Geometry: final body of the model. Coordinates: model frame, mm. A direction names the side the tool comes from. Coordinates: 2 decimals unless noted, no trailing zeros. Order: outer loops, then holes, each group sorted by start corner. A loop starts at its lowest first (then second) coordinate and runs counter-clockwise, first axis right, second up. Notation, with made-up numbers: M 1,51.5 L 19,51.5 A29 ccw 19,81.5 Z; hole C 0,-9 d11. An arc over 180 degrees is marked long. Use CSV: the item, a comma, the result in double quotes. Start each with the question number.
Q1. Access query for faces 1 (the face through (36.1, 4, -8)), 2 (the face through (40, 4, -3.1)), 3 (the face through (41, 3.3, -8)). Directions: +Z, -Z, +X, -X, +Y, -Y. A direction counts if a zero-diameter tool reaches every point of the face in a straight line with its end or side. Return the directions, or none.
Q2. First-contact query: P1, Ø0.5, axis at x = 41, y = 4, coming from the -Z side; P2, Ø6, axis at x = 14, z = -13.5, coming from the +Y side; P3, Ø1.1, axis at x = 40, y = 3.5, coming from the +Z side. Flat tips, straight axial feed; report the tip coordinate or a pass-through.
Q3. Section query C-C, the plane y = 3.85. Output: boundary loops of the cut face in (x, z), and give its area (3 significant figures).
Q4. Section query B-B, the plane x = 29. Output: boundary loops of the cut face in (y, z), and give its area (3 significant figures).
Q5. Section query A-A, the plane z = -8.5. Output: boundary loops of the cut face in (x, y).
Q6. Ray query, probe 1 along X at (y, z) = (0.2, -3.5); probe 2 along Y at (x, z) = (3, -5); probe 3 along Y at (x, z) = (39.5, -12.5). Return the intervals inside material, ascending.
from build123d import *

# Parameters (mm, degrees)
SKETCH_1_W      = 38.6
SKETCH_1_H      = 16.2
EXTRUDE_1_DEPTH = 3.3
SKETCH_2_W      = 2.5
SKETCH_2_H      = 10
EXTRUDE_2_DEPTH = 1
SKETCH_3_W      = 10
SKETCH_3_H      = 1
EXTRUDE_3_DEPTH = 5.5


with BuildPart() as part:
    # 草图1 → 凸台-拉伸1 (new body)
    with BuildSketch(Plane(origin=(0, 0, 0), x_dir=(1, 0, 0), z_dir=(0, 1, 0))):
        with Locations((19.3, 8.1)):
            Rectangle(SKETCH_1_W, SKETCH_1_H)
    extrude(amount=EXTRUDE_1_DEPTH)

    # 草图2 → 凸台-拉伸2 (add)
    with BuildSketch(Plane(origin=(0, 3.3, 0), x_dir=(1, 0, 0), z_dir=(0, 1, 0))):
        with Locations((37.35, 8.1)):
            Rectangle(SKETCH_2_W, SKETCH_2_H)
    extrude(amount=EXTRUDE_2_DEPTH)

    # 草图3 → 凸台-拉伸3 (add)
    with BuildSketch(Plane(origin=(38.6, 0, 0), x_dir=(0, 0, -1), z_dir=(1, 0, 0))):
        with Locations((8.1, 3.8)):
            Rectangle(SKETCH_3_W, SKETCH_3_H)
    extrude(amount=EXTRUDE_3_DEPTH)


solid = part.part
Responses:
1,face 1,"+Z, -Z, -X, +Y"
1,face 2,"+Z, +X, -X, +Y"
1,face 3,"+Z, -Z, +X, -Y"
2,P1,"stops at z = -13.1"
2,P2,"stops at y = 3.3"
2,P3,"stops at z = -3.1"
3,outline,"M 36.1,-13.1 L 44.1,-13.1 L 44.1,-3.1 L 36.1,-3.1 Z"
3,area,"80.0 mm²"
4,outline,"M 0,-16.2 L 3.3,-16.2 L 3.3,0 L 0,0 Z"
4,area,"53.5 mm²"
5,outline,"M 0,0 L 38.6,0 L 38.6,3.3 L 44.1,3.3 L 44.1,4.3 L 36.1,4.3 L 36.1,3.3 L 0,3.3 Z"
6,probe 1,"x = 0 to 38.6"
6,probe 2,"y = 0 to 3.3"
6,probe 3,"y = 3.3 to 4.3"
